from build123d import *

# Parameters (mm, degrees)
CBORE_FOR_M6_HEX_SOCKET_HEAD_CAP_SCREW1_D           = 6.6
CBORE_FOR_M6_HEX_SOCKET_HEAD_CAP_SCREW1_CBORE_D     = 11
CBORE_FOR_M6_HEX_SOCKET_HEAD_CAP_SCREW1_CBORE_DEPTH = 5
CIRPATTERN1_COUNT                                   = 6


with BuildPart() as part:
    # Sketch1 → Revolve1 (revolve)
    with BuildSketch(Plane(origin=(0, 0, 0), x_dir=(0, 0, -1), z_dir=(1, 0, 0)), mode=Mode.PRIVATE) as revolve1_sk:
        with BuildLine():
            Line((9, 24.5), (11, 24.5))
            Line((11, 24.5), (17, 30.5))
            Line((17, 30.5), (17, 54))
            Line((17, 54), (16, 55))
            Line((16, 55), (1, 55))
            Line((1, 55), (0, 54))
            Line((0, 54), (0, 36))
            Line((0, 36), (1, 35))
            Line((1, 35), (8, 35))
            ThreePointArc((8, 35), (8.707106781, 34.707106781), (9, 34))
            Line((9, 34), (9, 24.5))
        make_face()
    revolve(revolve1_sk.sketch.rotate(Axis((0, 0, 0), (0, 0, -1)), 90), axis=Axis((0, 0, 0), (0, 0, -1)))

    # CBORE for M6 Hex Socket Head Cap Screw1 (through all)
    with Locations(Plane.XY):
        with Locations((0, 45)):
            cbore_for_m6_hex_socket_head_cap_screw1 = CounterBoreHole(CBORE_FOR_M6_HEX_SOCKET_HEAD_CAP_SCREW1_D / 2, CBORE_FOR_M6_HEX_SOCKET_HEAD_CAP_SCREW1_CBORE_D / 2, CBORE_FOR_M6_HEX_SOCKET_HEAD_CAP_SCREW1_CBORE_DEPTH)

    # CirPattern1: CBORE for M6 Hex Socket Head Cap Screw1 ×6 about axis
    cirpattern1_axis = Axis((0, 0, 0), (0, 0, 1))
    for i in range(1, CIRPATTERN1_COUNT):
        add(cbore_for_m6_hex_socket_head_cap_screw1.rotate(cirpattern1_axis, i * 360 / CIRPATTERN1_COUNT), mode=Mode.SUBTRACT)


solid = part.part
Geometry: final body of the model. Coordinates: model frame, mm. A direction names the side the tool comes from. Coordinates: 2 decimals unless noted, no trailing zeros. Order: outer loops, then holes, each group sorted by start corner. A loop starts at its lowest first (then second) coordinate and runs counter-clockwise, first axis right, second up.
1) Draft query along X for faces 3 (the flat face through (-23, 23, -17)), 4 (the flat face through (-37, 26, -5)), 5 (the cylindrical face through (25.379, 48.794, -8.395)). Return one class per face: released by +X, released by -X, zero draft, split by the parting line, or undercut.
Result sheet:
face 3: zero draft
face 4: undercut
face 5: split by the parting line
2) Section B-B (x = 0). Give the number of separate pieces and of enclosed holes in the cut face, then the cut area to 3 significant figures.
Result sheet:
separate pieces: 4
enclosed holes: 0
area: 541 mm2
3) Set-up query: faces 1 (the cylindrical face through (-0.43, -48.27, -11.08)), 2 (the cylindrical face through (-0.716, 50.453, -2.465)). Return all of +Z, -Z, +X, -X, +Y, -Y with unobstructed straight access to the full face (end or side cutting, diameter ignored); none if empty.
Result sheet:
face 1: +Z, -Z
face 2: +Z
4) Ray query, probe 1 along Y at (x, z) = (-38.5, -12); probe 2 along X at (y, z) = (26.5, -2); probe 3 along Y at (x, z) = (-37, -10.5). Return the intervals inside material, ascending.
Result sheet:
probe 1: y = -39.28 to -25.77, -19.23 to 19.23, 25.77 to 39.28
probe 2: x = -48.19 to -42.75, -35.2 to -22.86, 22.86 to 35.2, 42.75 to 48.19
probe 3: y = -40.69 to -25.15, -19.85 to 19.85, 25.15 to 40.69
5) Section A-A (y = 0). Return loops of the section in (x, z), then the cut area to 3 significant figures.
Result sheet:
outline: (-55, -16) - (-54, -17) - (-30.5, -17) - (-24.5, -11) - (-24.5, -9) - (-34, -9) arc R1 cw to (-35, -8) - (-35, -1) - (-36, 0) - (-54, 0) - (-55, -1) - close; (24.5, -11) - (30.5, -17) - (54, -17) - (55, -16) - (55, -1) - (54, 0) - (36, 0) - (35, -1) - (35, -8) arc R1 cw to (34, -9) - (24.5, -9) - close
area: 809 mm2
6) First-contact query: P1, Ø3, axis at y = -25.5, z = -7.5, coming from the -X side; P2, Ø8, axis at x = -44, z = -12.5, coming from the +Y side; P3, Ø10, axis at x = 27, y = 9, coming from the -Z side; P4, Ø3.5, axis at x = 38, y = 20.5, coming from the +Z side. Flat tips, straight axial feed; report the tip coordinate or a pass-through.
Result sheet:
P1: stops at x = -49.49
P2: stops at y = 37.75
P3: stops at z = -17
P4: stops at z = -5
